For this review, take the finished solid that the model builds, in its own axes (mm). A direction names the side the tool comes from. Round coordinates to 2 decimals unless told otherwise and drop trailing zeros.
from build123d import *

# Parameters (mm, degrees)
F1_DEPTH = 27
F3_R     = 91.9406887246
F4_DEPTH = 6.5
F6_DEPTH = 43.7
F8_DEPTH = 96
F9_R     = 1


with BuildPart() as f1:
    # F0 (on Right) → F1 (new body)
    with BuildSketch(Plane.YZ):
        Polygon((10.3527618041, 38.6370330516), (0, 0), (80.6664137916, 0), (21.2226228125, 38.6370330516), align=None)
    extrude(amount=F1_DEPTH)

    # F3 (on offset) → F4 (cut)
    with BuildSketch(Plane(origin=(0, 4.8296291314, -1.2940952255), x_dir=(1, 0, 0), z_dir=(0, -0.9659258263, 0.2588190451))):
        with Locations((13.5, 110)):
            Circle(F3_R)
    extrude(amount=-F4_DEPTH, mode=Mode.SUBTRACT)

    # F5 (on face) → F6 (cut)
    with BuildSketch(Plane(origin=(0, 0, 0), x_dir=(0, -1, 0), z_dir=(-1, 0, 0))):
        Polygon((-18.6758581549, 34.7778759897), (-12.6453930714, 27.8747328985), (-15.5291427062, 38.6370330516), (-10.3527618041, 38.6370330516), (-7.81576394, 29.168828124), (-5.5674631149, 30.5033978075), (-7.2772535495, 43.6117947102), (-16.111170873, 47.3163388669), align=None)
        Polygon((-15.5291427062, 38.6370330516), (-12.6453930714, 27.8747328985), (-7.81576394, 29.168828124), (-10.3527618041, 38.6370330516), align=None)
    extrude(amount=-F6_DEPTH, mode=Mode.SUBTRACT)

    # F7 (on Front) → F8 (cut)
    with BuildSketch(Plane.XZ):
        Polygon((21.458028581, 51.2392446399), (27, 0), (40.6126193702, -9.302303195), (49.8705804348, 59.140522033), align=None)
        Polygon((-22.2092997283, -20.874761045), (0, 0), (5.541971419, 51.2392446399), (-20.2254503965, 29.3827727437), align=None)
    extrude(amount=-F8_DEPTH, mode=Mode.SUBTRACT)

    # F9
    f9_edges = [f1.edges().sort_by_distance(p)[0] for p in [
        (2.880945, 19.042842, 26.636267),
        (13.5, 22.104798, 38.063641),
        (2.058457, 51.385606, 19.03182),
        (24.941543, 51.385606, 19.03182),
        (13.5, 80.666414, 0),
        (24.119055, 19.042842, 26.636267),
        (13.5, 15.782241, 14.467536),
        (24.580296, 11.170883, 22.371787),
        (27, 40.333207, 0),
        (25.265261, 12.838619, 16.038825),
        (23.915121, 10.230579, 28.521781),
        (25.422568, 3.907882, 14.584414),
        (13.5, 0, 0),
        (0, 40.333207, 0),
        (13.5, 7.815764, 29.168828),
        (1.577432, 3.907882, 14.584414),
        (13.5, 9.503723, 16.14986),
        (1.734739, 12.838619, 16.038825),
        (3.084879, 10.230579, 28.521781),
        (13.5, 12.645393, 27.874733),
        (2.419704, 11.170883, 22.371787),
    ]]
    fillet(f9_edges, radius=F9_R)


solid = f1.part
(1) For line 1 along Y through (x, z) = (19.5, 21); line 2 along Y through (x, z) = (21, 17.5); line 3 along Y through (x, z) = (6, 7), list the stretches that pass through material, from the lowest coordinate up.
Geometry check:
line 1: y = 5.63 to 10.8, 17.53 to 48.36
line 2: y = 4.69 to 9.87, 16.59 to 53.74
line 3: y = 1.88 to 69.9
(2) For faces 4 (the face through (13.366, 10.251, 28.516)), 5 (the face through (13.348, 12.613, 15.317)), 6 (the face through (13, 39, 0)), 7 (the face through (3.325, 10.128, 28.29)), 8 (the face through (23.884, 19.239, 26.244)), list the 3-axis set-ups (+Z, -Z, +X, -X, +Y, -Y) from which the entire face can be reached by the end or side of a thin tool; tool diameter is ignored.
Geometry check:
face 4: +Z, +X, -X
face 5: none
face 6: -Z, +X, -X, +Y, -Y
face 7: +Z, -X
face 8: +Z, +X
(3) Mouldability with a two-part tool opening along Z and no side actions: class faces 1 (the face through (13.4, 11.1, 22.1)), 2 (the face through (13.673, 78.246, 0.699)), 3 (the face through (13.38, 22.369, 37.413)) as pulls with the +Z half, pulls with the -Z half, needs draft (parallel to the pull), parting line crosses it, or undercut.
Geometry check:
face 1: undercut
face 2: parting line crosses it
face 3: pulls with the +Z half
(4) For pin 1 Ø6 at (x, y) = (14.5, 12.5) entering from +Z; pin 2 Ø12 at (y, z) = (26.5, 11.5) entering from -X; pin 3 Ø12 at (y, z) = (24, 8.5) entering from -X, all flat-tipped, find the tip position at first contact; note any pin that passes through.
Geometry check:
pin 1: stops at z = 28.72
pin 2: stops at x = 0.59
pin 3: stops at x = 0.27
